For this review, use the dimensioned drawing (mm, ordinates from the lowest corner) and the shaded views. Coordinates: 2 decimals unless noted, no trailing zeros. Loops run counter-clockwise (first coordinate to the right, second up) from the corner with the lowest first, then second, coordinate; pieces in that order, holes last.
1. Take a section at C-C, the plane z = 5. State the section outline as (x, y) points, then the cut area to 3 significant figures.
2. To check wall thickness, follow probe 1 along Y at (x, z) = (8.5, 21); probe 2 along Y at (x, z) = (11.35, 5); probe 3 along X at (y, z) = (8, 37). State the ranges of each line that lie inside material, in increasing order.
3. Clearance check with flat-ended pins moving along their axes: P1, Ø6, axis at x = 12, y = 24.5, coming from the +Z side; P2, Ø4, axis at x = 5.5, z = 23.5, coming from the -Y side; P3, Ø2, axis at x = 6.5, z = 26, coming from the -Y side. State where each tip first meets the part, or that it passes through.
4. Take a section at A-A, the plane z = 21. Count the separate pieces of the cut face and the enclosed holes in it, then the cut area to 3 significant figures.
5. Mouldability with a two-part tool opening along Z and no side actions: class the marked faces 1, 2 and 3 as pulls with the +Z half, pulls with the -Z half, needs draft (parallel to the pull), parting line crosses it, or undercut.
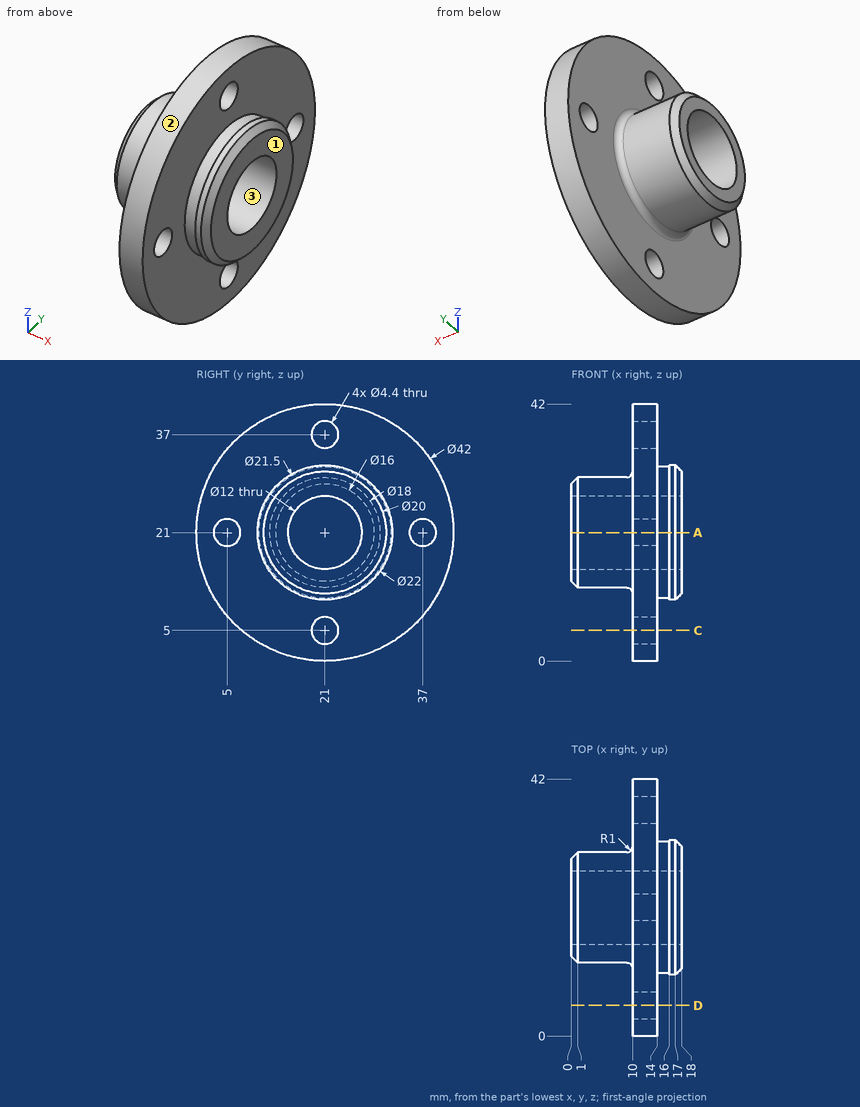
Results list:
1. outline: (10, 7.4) - (14, 7.4) - (14, 18.8) - (10, 18.8) - close; (10, 23.2) - (14, 23.2) - (14, 34.6) - (10, 34.6) - close
1. area: 91.2 mm2
2. probe 1: y = 12 to 15, 27 to 30
2. probe 2: y = 7.4 to 18.8, 23.2 to 34.6
2. probe 3: x = 10 to 14
3. P1: stops at z = 41.99
3. P2: stops at y = 12.01
3. P3: stops at y = 12.94
4. separate pieces: 4
4. enclosed holes: 0
4. area: 182 mm2
5. face 1: needs draft
5. face 2: parting line crosses it
5. face 3: undercut
